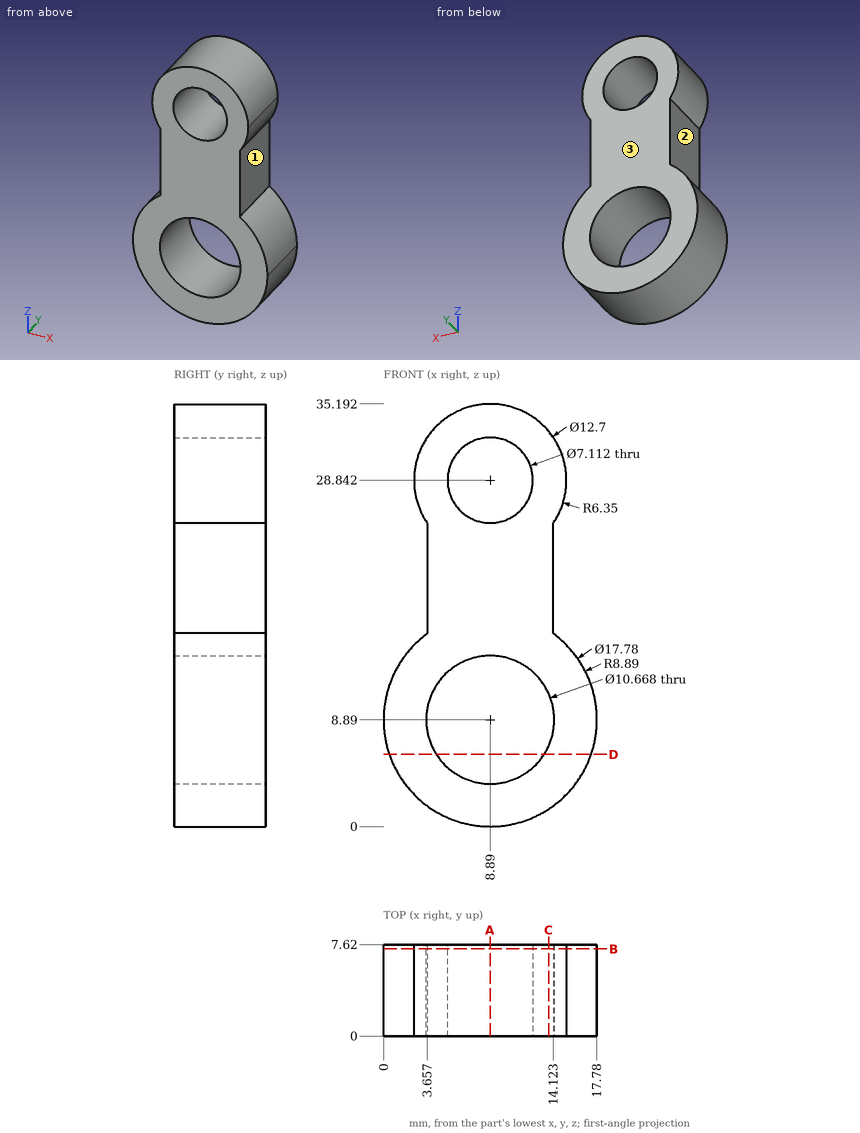
The figure shows three views and two pictorial views of one solid part (mm, origin at its lowest corner). Answer the questions. A direction names the side the tool comes from. Coordinates: 2 decimals unless noted, no trailing zeros. Loops run counter-clockwise (first coordinate to the right, second up) from the corner with the lowest first, then second, coordinate; pieces in that order, holes last. Notation, with made-up numbers: M 23,-8 L 29,-8 A13 ccw 29,4 Z; hole C 32.5,82 d11. An arc over 180 degrees is marked long. Answer as CSV lines item,"result". Start each with the question number.
(1) Find the intervals of material crossed by L1, parallel to Z at x = 8.75, y = 1.75 (1 decimal); L2, parallel to X at y = 3.25, z = 29; L3, parallel to Z at x = 6.5, y = 3 (1 decimal), in increasing order. Write a range as [from, to].
(2) The part is cut by section D-D (z = 6). Give the vertices of the cut face in (x, y).
(3) For the marked faces 1, 2 and 3, determine the directions among +Z, -Z, +X, -X, +Y, -Y from which every point of the face is accessible in a straight line to the end or side of a thin tool.
(4) The part is cut by section A-A (x = 8.89). Give the vertices of the cut face in (y, z) (1 decimal), and give its area (3 significant figures).
(5) The part is cut by section C-C (x = 13.75). Give the vertices of the cut face in (y, z), and give its area (3 significant figures).
(6) Given pin 1 (6.5 mm diameter, centred on x = 8.89, z = 8.89, fed in from -Y); pin 2 (1.5 mm diameter, centred on x = 2, y = 1, fed in from -Z); pin 3 (3 mm diameter, centred on y = 1, z = 14.5, fed in from -X); pin 4 (3 mm diameter, centred on y = 1, z = 22.5, fed in from -X), each flat-ended and moving along its own axis, determine where each tip first touches the part or whether it passes through.
(7) The part is cut by section B-B (y = 7.25). State how many separate pieces and enclosed holes the cut face has.
Determined:
1,L1,"[0, 3.6], [14.2, 25.3], [32.4, 35.2]"
1,L2,"[2.54, 5.34], [12.44, 15.24]"
1,L3,"[0.3, 4.1], [13.7, 26.2], [31.5, 34.7]"
2,outline,"M 0.48,0 L 4.41,0 L 4.41,7.62 L 0.48,7.62 Z; M 13.37,0 L 17.3,0 L 17.3,7.62 L 13.37,7.62 Z"
3,face 1,"+X, +Y, -Y"
3,face 2,"-X, +Y, -Y"
3,face 3,"+Z, -Z, +X, -X, +Y"
4,outline,"M 0,0 L 7.6,0 L 7.6,3.6 L 0,3.6 Z; M 0,14.2 L 7.6,14.2 L 7.6,25.3 L 0,25.3 Z; M 0,32.4 L 7.6,32.4 L 7.6,35.2 L 0,35.2 Z"
4,area,"133 mm2"
5,outline,"M 0,1.45 L 7.62,1.45 L 7.62,6.69 L 0,6.69 Z; M 0,11.09 L 7.62,11.09 L 7.62,32.93 L 0,32.93 Z"
5,area,"206 mm2"
6,pin 1,"through"
6,pin 2,"z = 2.46"
6,pin 3,"x = 1.01"
6,pin 4,"x = 3.66"
7,separate pieces,"1"
7,enclosed holes,"2"
